The listing builds one solid part. Answer for the finished solid, in the listing's coordinates (mm). A direction names the side the tool comes from. Coordinates: 2 decimals unless noted, no trailing zeros. Loops run counter-clockwise (first coordinate to the right, second up) from the corner with the lowest first, then second, coordinate; pieces in that order, holes last. Notation, with made-up numbers: (62, 21) - (83, 21) arc R19 ccw to (83, 30) - close; hole circle Ø5 at (10.5, -9.5). An arc over 180 degrees is marked (long way). Put each result on its own line as item: value.
Autodesk Inventor part; units mm, degrees
ref_plane "YZ Plane" through (0, 0, 0) normal (1, 0, 0) x (0, 1, 0)
ref_plane "XZ Plane" through (0, 0, 0) normal (0, 1, 0) x (-1, 0, 0)
ref_plane "XY Plane" through (0, 0, 0) normal (0, 0, 1) x (1, 0, 0)
sketch "Sketch1" plane through (0, 0, 0) normal (0, 0, 1) x (1, 0, 0)
  line L0 (6.3387, 0) -> (6.3387, 31.7461)
  line L1 (0, 31.7461) -> (3.15, 36.0063)
  line L2 (3.15, 36.0063) -> (6.3387, 31.7461)
  line L3 (6.3387, 0) -> (0, 0)
  line L4 (0, 0) -> (0, 31.7461)
extrude "Extrusion1" add sketch "Sketch1" along normal blind 5.08
sketch "Sketch2" plane through (0, 0, 0) normal (0, 0, -1) x (-1, 0, 0)
  line L0 (0, 0) -> (-6.3387, 0)
  line L1 (0, 31.7461) -> (0, 0)
  line L2 (-6.3387, 0) -> (0, 0)
  line L3 (0, 0) -> (0, 3.1419)
  line L4 (0, 3.1419) -> (-6.3387, 3.1419)
  line L5 (-6.3387, 3.1419) -> (-6.3387, 0)
extrude "Extrusion2" add sketch "Sketch2" along normal blind 1.27
properties part number "Needle"
1) The part is cut by section B-B (z = 3.75). Give the vertices of the cut face in (x, y).
Found:
outline: (0, 0) - (6.34, 0) - (6.34, 31.75) - (3.15, 36.01) - (0, 31.75) - close
2) The part is cut by section C-C (x = 2.75). Give the vertices of the cut face in (y, z).
Found:
outline: (0, -1.27) - (3.14, -1.27) - (3.14, 0) - (35.47, 0) - (35.47, 5.08) - (0, 5.08) - close
3) The part is cut by section A-A (y = 17). Give the vertices of the cut face in (x, z).
Found:
outline: (0, 0) - (6.34, 0) - (6.34, 5.08) - (0, 5.08) - close
4) Straight lines are drawn through the part: L1, parallel to Y at x = 5.5, z = -0.5; L2, parallel to Z at x = 1.25, y = 6; L3, parallel to Y at x = 1.5, z = 3.5. For each, find the intervals that lie inside material, in ascending order. Write a range as [from, to].
Found:
L1: y = [0, 3.14]
L2: z = [0, 5.08]
L3: y = [0, 33.77]
5) Each of these flat-tipped pins is pushed along its axis until it touches: pin 1 (1 mm diameter, centred on x = 3.5, z = -1, fed in from +Y); pin 2 (3 mm diameter, centred on x = 4.5, y = 12, fed in from -Z); pin 3 (2 mm diameter, centred on x = 2, z = 4, fed in from +Y). Where does it stop, or does it pass through?
Found:
pin 1: stops at y = 3.14
pin 2: stops at z = 0
pin 3: stops at y = 35.8
6) For faces 1 (the face through (3, 20, 0)), 2 (the face through (3, 0, 2)), determine the directions among +Z, -Z, +X, -X, +Y, -Y from which every point of the face is accessible in a straight line to the end or side of a thin tool.
Found:
face 1: -Z, +X, -X, +Y
face 2: +Z, -Z, +X, -X, -Y
7) The part is cut by section D-D (x = 4.75). Give the vertices of the cut face in (y, z), and give its area (3 significant figures).
Found:
outline: (0, -1.27) - (3.14, -1.27) - (3.14, 0) - (33.87, 0) - (33.87, 5.08) - (0, 5.08) - close
area: 176 mm^2
